```python
from build123d import *

# Parameters (mm, degrees)
SKETCH1_R           = 1.8
BOSS_EXTRUDE1_DEPTH = 15
SKETCH2_R           = 3
BOSS_EXTRUDE2_DEPTH = 2


with BuildPart() as part:
    # Sketch1 → Boss-Extrude1 (new body)
    with BuildSketch(Plane(origin=(0, 0, 0), x_dir=(1, 0, 0), z_dir=(0, 1, 0))):
        with Locations(Location((0, 0, 0), (0, 0, 270))):
            Circle(SKETCH1_R)
    extrude(amount=BOSS_EXTRUDE1_DEPTH)

    # Sketch2 → Boss-Extrude2 (add)
    with BuildSketch(Plane(origin=(0, 15, 0), x_dir=(1, 0, 0), z_dir=(0, 1, 0))):
        with Locations(Location((0, 0, 0), (0, 0, 270))):
            Circle(SKETCH2_R)
    extrude(amount=BOSS_EXTRUDE2_DEPTH)

    # Sketch3 → Revolve1 (revolve)
    with BuildSketch(Plane.XY):
        with BuildLine():
            Line((0, 17), (-3, 17))
            add(Edge.make_bspline(
                [(-3, 17), (-2.027477475, 17.462743373), (-0.971060037, 17.5), (0, 17.5)],
                knots=[0, 0, 0, 0, 1, 1, 1, 1], degree=3))
            Line((0, 17.5), (0, 17))
        make_face()
    revolve(axis=Axis((0, 17, 0), (0, 1, 0)))

    # Sketch4 → Revolve3 (revolve)
    with BuildSketch(Plane.XY, mode=Mode.PRIVATE) as revolve3_sk:
        Polygon((0, 0), (1.500760402, 0), (0.125, -14.5), (0, -14.5), align=None)
    revolve(revolve3_sk.sketch.rotate(Axis((0, 0, 0), (0, -1, 0)), 180), axis=Axis((0, 0, 0), (0, -1, 0)))


solid = part.part
```
Verification items for the finished model (mm, model axes). A direction names the side the tool comes from. Give positions to 0.01 mm unless a question says otherwise; leave off trailing zeros. Order: outer loops, then holes, each group sorted by start corner. A loop starts at its lowest first (then second) coordinate and runs counter-clockwise, first axis right, second up. Notation, with made-up numbers: M 89.25,-25 L 107.25,-25 A34 ccw 107.25,7 Z; hole C 14,45.25 d4. An arc over 180 degrees is marked long. Return JSON: item names as keys, results as strings. Group by question number.
1) Scan lines: line 1 (X direction, y = 6, z = 1); line 2 (Z direction, x = -0.25, y = 2); line 3 (Y direction, x = -1.25, z = 1.25). Record each from-to range of solid material in increasing order.
2) Section check A-A on y = 9.5. Record the cut outline in (x, z), and give its area (3 significant figures).
3) Access from +Z, -Z, +X, -X, +Y, -Y to the whole of each face (thin tool, end or side, straight path). Record for faces 1 (the face through (-0.689, 7.395, 1.663)), 2 (the face through (0.9, 15.99, 2.86)).
4) Go/stop test with flat-tipped pins: pin 1 Ø1 at (x, y) = (0.5, -1) entering from +Z; pin 2 Ø2 at (x, y) = (-0.5, -9.5) entering from -Z; pin 3 Ø1.5 at (x, z) = (0, 1.5) entering from +Y. Record where each tip stops, or that it passes through.
5) Section check B-B on y = -4.5. Record the cut outline in (x, z), and give its area (3 significant figures).
Answer block:
{
 "1": {"line 1": "x = -1.5 to 1.5", "line 2": "z = -1.78 to 1.78", "line 3": "y = 0 to 17.38"},
 "2": {"outline": "C 0,0 d3.6", "area": "10.2 mm^2"},
 "3": {"face 1": "-Y", "face 2": "+Y, -Y"},
 "4": {"pin 1": "stops at z = 1.43", "pin 2": "stops at z = -0.68", "pin 3": "stops at y = 17.49"},
 "5": {"outline": "C 0,0 d2.15", "area": "3.62 mm^2"}
}
